Verification items for the finished model (mm, model axes). Round coordinates to 2 decimals unless told otherwise and drop trailing zeros. Order: outer loops, then holes, each group sorted by start corner. A loop starts at its lowest first (then second) coordinate and runs counter-clockwise, first axis right, second up. Notation, with made-up numbers: (65, -28.75) -> (108, -28.75) arc R14 ccw to (108, -3.75) -> close; hole circle Ø9 at (86.25, 18). An arc over 180 degrees is marked (long way). Return JSON: item names as keys, results as strings. Group by question number.
Item 1: Sectioned sample at A-A on z = 7.5. Record the cut outline in (x, y), plus the area to 3 significant figures.
Item 2: Sectioned sample at C-C on x = 37. Record the cut outline in (y, z), plus the area to 3 significant figures.
Item 3: Scan lines: probe 1 along Y at (x, z) = (27.5, 2.75); probe 2 along X at (y, z) = (11, 6.75); probe 3 along X at (y, z) = (12.5, 9.5). Record each from-to range of solid material in increasing order. Write a range as from..to.
Item 4: Depth check by flat-ended pin: pin 1 Ø3 at (y, z) = (-15.5, 2) entering from -X; pin 2 Ø2 at (x, z) = (36.5, 6.5) entering from +Y. Enter the tip coordinate at first touch or a pass-through.
Item 5: Sectioned sample at B-B on y = -16. Record the cut outline in (x, z), plus the area to 3 significant figures.
Autodesk Inventor part; units mm, degrees
ref_plane "YZ Plane" through (0, 0, 0) normal (1, 0, 0) x (0, 1, 0)
ref_plane "XZ Plane" through (0, 0, 0) normal (0, 1, 0) x (-1, 0, 0)
ref_plane "XY Plane" through (0, 0, 0) normal (0, 0, 1) x (1, 0, 0)
sketch "Sketch1" plane through (0, 0, 0) normal (0, 0, 1) x (1, 0, 0)
  circle A0 centre (40, 19.5) radius 1.85
  circle A1 centre (-57.5, -20.4606) radius 1.85
  circle A2 centre (-57.5, 19.5) radius 1.85
  circle A3 centre (57.5, -20.4606) radius 1.85
  line L0 (63, 25) -> (-63, 25)
  line L1 (-63, 25) -> (-63, -25)
  line L2 (-63, -25) -> (63, -25)
  line L3 (63, -25) -> (63, 25)
  line L4 (50, -20) -> (-50, -20)
  line L5 (-50, -20) -> (-50, 20)
  line L6 (-50, 20) -> (50, 20)
  line L7 (50, 20) -> (50, -20)
  line L8 (50, -20) -> (-50, 20) construction
  line L9 (-50, -20) -> (50, 20) construction
  point P0 (0, 0)
  dimension "d0" = 40
  dimension "d1" = 100
extrude "Extrusion1" add sketch "Sketch1" along normal blind 10 contours A0 L6 | A0 L6 L7 L4 L5 picked at (39.6393, 19.3331)
chamfer "Chamfer1" distance 20 angle 45 1 edges at (50, 20, 5)
fillet "Fillet1" radius 10 5 edges at (-50, 20, 5) (30, 20, 5) (50, 0, 5) (50, -20, 5) (-50, -20, 5)
properties part number "Frame_Foot_Flex" material "Rubber, Silicone"
Recorded:
{
 "1": {"outline": "(-50, -10) arc R10 ccw to (-40, -20) -> (40, -20) arc R10 ccw to (50, -10) -> (50, -4.14) arc R10 ccw to (47.07, 2.93) -> (32.93, 17.07) arc R10 ccw to (25.86, 20) -> (-40, 20) arc R10 ccw to (-50, 10) -> close", "area": "3,730 mm²"},
 "2": {"outline": "(-20, 0) -> (13, 0) -> (13, 10) -> (-20, 10) -> close", "area": "330 mm²"},
 "3": {"probe 1": "-20..19.86", "probe 2": "-49.95..39", "probe 3": "-49.68..37.5"},
 "4": {"pin 1": "x = -49.17", "pin 2": "y = 14.5"},
 "5": {"outline": "(-48, 0) -> (48, 0) -> (48, 10) -> (-48, 10) -> close", "area": "960 mm²"}
}
